Input: part model. Units: mm. Frame: model coordinates. A direction names the side the tool comes from. Coordinates: 2 decimals unless noted, no trailing zeros. Loops run counter-clockwise (first coordinate to the right, second up) from the corner with the lowest first, then second, coordinate; pieces in that order, holes last. Notation, with made-up numbers: (53.5, 70.5) -> (94.5, 70.5) arc R16 ccw to (94.5, 85.5) -> close; hole circle Ø6 at (3, -2). An arc over 180 degrees is marked (long way). Answer as a JSON object with one key per item and string values.
Autodesk Fusion 360 part; units mm, degrees
sketch "Sketch1" plane through (0, 0, 0) normal (0, 0, 1) x (1, 0, 0)
  line L0 (0, 0) -> (63.5, 0)
  line L1 (63.5, 0) -> (63.5, 19.05)
  line L2 (63.5, 19.05) -> (0, 19.05)
  line L3 (0, 19.05) -> (0, 0)
  dimension "d1" = 63.5
  dimension "d2" = 19.05
extrude "Extrude1" add sketch "Sketch1" along normal blind 6.35
sketch "Sketch2" plane through (0, 0, 6.35) normal (0, 0, 1) x (-1, 0, 0)
  line L0 (0, -19.05) -> (0, 0)
  line L1 (0, 0) -> (-63.5, 0)
  line L2 (-63.5, 0) -> (-63.5, -19.05)
  line L3 (-63.5, -19.05) -> (0, -19.05)
  line L4 (0, 0) -> (0, -9.525)
  line L5 (0, -19.05) -> (-9.2075, -19.05)
  circle A0 centre (-9.2075, -9.4653) radius 4.0005
  line L6 (0, -19.05) -> (-18.415, -19.05)
  line L7 (-1.154, -19.05) -> (-2.7137, -19.7589)
  line L8 (0, -19.05) -> (-24.765, -19.05)
  line L9 (-24.765, -19.05) -> (-18.415, -19.05)
  line L10 (-18.415, -19.05) -> (-18.415, 0)
  line L11 (-18.415, 0) -> (-24.765, 0)
  line L12 (-24.765, 0) -> (-24.765, -19.05)
  line L13 (-24.765, -19.05) -> (-38.735, -19.05)
  line L14 (-63.5, -19.05) -> (-54.2925, -19.05)
  line L15 (-63.5, -19.05) -> (-45.085, -19.05)
  line L16 (-63.5, 0) -> (-63.5, -9.525)
  circle A1 centre (-54.2925, -9.6525) radius 4.0005
  line L17 (-38.735, -19.05) -> (-38.735, 0)
  line L18 (-45.085, -19.05) -> (-45.085, 0)
  line L19 (-45.085, -19.05) -> (-38.735, -19.05)
  line L20 (-38.735, -19.05) -> (-38.735, 0)
  line L21 (-38.735, 0) -> (-45.085, 0)
  line L22 (-45.085, 0) -> (-45.085, -19.05)
  dimension "d5" = 9.525
  dimension "d6" = 9.2075
  dimension "d7" = 8.001
  dimension "d8" = 18.415
  dimension "d9" = 24.765
  dimension "d10" = 6.35
  dimension "d11" = 19.05
  dimension "d12" = 13.97
  dimension "d13" = 9.2075
  dimension "d14" = 18.415
  dimension "d15" = 9.525
  dimension "d16" = 8.001
extrude "Extrude2" cut sketch "Sketch2" against normal blind 1.27 contours L1 L3 L8 L9 L10 L11 L12 | L1 L3 L17 L18 L19 L20 L21 L22
1. Mould query, pull axis X, two halves, no side actions, for faces 1 (the face through (0, 10, 3)), 2 (the face through (63.5, 9, 3)), 3 (the face through (9, 10, 6.35)), 4 (the face through (22, 9, 5.08)). Classes: pulls with the +X half, pulls with the -X half, needs draft (parallel to the pull), parting line crosses it, or undercut.
Reply:
{"face 1": "pulls with the -X half", "face 2": "pulls with the +X half", "face 3": "needs draft", "face 4": "undercut"}
2. Section query B-B (x = 43.5). Return loops of the section in (y, z).
Reply:
{"outline": "(0, 0) -> (19.05, 0) -> (19.05, 5.08) -> (0, 5.08) -> close"}
3. Section query A-A (y = 5.5). Return loops of the section in (x, z) (3 decimals).
Reply:
{"outline": "(0, 0) -> (63.5, 0) -> (63.5, 6.35) -> (45.085, 6.35) -> (45.085, 5.08) -> (38.735, 5.08) -> (38.735, 6.35) -> (24.765, 6.35) -> (24.765, 5.08) -> (18.415, 5.08) -> (18.415, 6.35) -> (0, 6.35) -> close"}
4. Pin query (flat end, axial travel): P1, Ø4, axis at x = 42, y = 2.5, coming from the +Z side. Return the tip coordinate at first contact, or that it passes through.
Reply:
{"P1": "stops at z = 5.08"}
5. Access query for faces 5 (the face through (24.765, 9, 6)), 6 (the face through (54, 10, 6.35)). Directions: +Z, -Z, +X, -X, +Y, -Y. A direction counts if a zero-diameter tool reaches every point of the face in a straight line with its end or side. Return the directions, or none.
Reply:
{"face 5": "+Z, +Y, -Y", "face 6": "+Z, +X, -X, +Y, -Y"}
6. Line query: line 1 along X through (y, z) = (17.5, 6) (3 decimals); line 2 along Z through (x, y) = (20.5, 2.25). Output: solid intervals per line, ascending.
Reply:
{"line 1": "x = 0 to 18.415, 24.765 to 38.735, 45.085 to 63.5", "line 2": "z = 0 to 5.08"}
